```python
from build123d import *

# Parameters (mm, degrees)
SKETCH1_R           = 9.6
SKETCH1_R_2         = 4.2
BOSS_EXTRUDE1_DEPTH = 2
SKETCH4_W           = 58
SKETCH4_H           = 57.7
SKETCH4_R           = 2
SKETCH4_R_2         = 9.6
BOSS_EXTRUDE3_DEPTH = 2
SKETCH5_R           = 2
CUT_EXTRUDE1_DEPTH  = 4
SKETCH6_W           = 43
SKETCH6_H           = 57.7
SKETCH6_R           = 3.75
SKETCH6_R_2         = 9.6
SKETCH6_R_3         = 2
BOSS_EXTRUDE4_DEPTH = 5
CUT_EXTRUDE2_DEPTH  = 48.972101267
BOSS_EXTRUDE5_DEPTH = 6
BOSS_EXTRUDE6_DEPTH = 1.5


with BuildPart() as part:
    # Sketch1 → Boss-Extrude1 (new body)
    with BuildSketch(Plane.XY):
        with BuildLine():
            Line((38, 28.85), (20, 28.85))
            Line((20, 28.85), (20, 21.79369023))
            Line((20, 21.79369023), (17.201699017, 17.757141063))
            ThreePointArc((17.201699017, 17.757141063), (12.496432266, 16.141438171), (9.55, 20.15))
            Line((9.55, 20.15), (9.55, 28.85))
            Line((9.55, 28.85), (-9.55, 28.85))
            Line((-9.55, 28.85), (-9.55, 20.15))
            ThreePointArc((-9.55, 20.15), (-12.496432266, 16.141438171), (-17.201699017, 17.757141063))
            Line((-17.201699017, 17.757141063), (-20, 21.79369023))
            Line((-20, 21.79369023), (-20, -16.371914064))
            Line((-20, -16.371914064), (-16.312, -16.371914064))
            Line((-16.312, -16.371914064), (-12.349992933, -13.321914064))
            ThreePointArc((-12.349992933, -13.321914064), (-6.459906996, -14.088), (-7.225992933, -19.978085936))
            Line((-7.225992933, -19.978085936), (-11.188, -23.028085936))
            ThreePointArc((-11.188, -23.028085936), (-12.396848296, -23.676050863), (-13.75, -23.9))
            Line((-13.75, -23.9), (-20, -23.9))
            Line((-20, -23.9), (-20, -28.85))
            Line((-20, -28.85), (9.55, -28.85))
            Line((9.55, -28.85), (9.55, -19.7))
            ThreePointArc((9.55, -19.7), (12.496432266, -15.691438171), (17.201699017, -17.307141063))
            Line((17.201699017, -17.307141063), (20, -21.34369023))
            Line((20, -21.34369023), (20, -28.85))
            Line((20, -28.85), (38, -28.85))
            Line((38, -28.85), (38, 28.85))
        make_face()
        with Locations((0, 8.8)):
            Circle(SKETCH1_R, mode=Mode.SUBTRACT)
        with Locations((-5.725, -6.1)):
            Circle(SKETCH1_R_2, mode=Mode.SUBTRACT)
        with Locations((5.725, -6.1)):
            Circle(SKETCH1_R_2, mode=Mode.SUBTRACT)
    extrude(amount=BOSS_EXTRUDE1_DEPTH)

    # Sketch4 → Boss-Extrude3 (add)
    with BuildSketch(Plane.XY.offset(2)):
        with Locations((9, 0)):
            Rectangle(SKETCH4_W, SKETCH4_H)
        with Locations((13.75, -19.7)):
            Circle(SKETCH4_R, mode=Mode.SUBTRACT)
        with Locations((-13.75, 20.15)):
            Circle(SKETCH4_R, mode=Mode.SUBTRACT)
        with Locations((13.75, 20.15)):
            Circle(SKETCH4_R, mode=Mode.SUBTRACT)
        with Locations((-13.75, -19.7)):
            Circle(SKETCH4_R, mode=Mode.SUBTRACT)
        with Locations((0, 8.8)):
            Circle(SKETCH4_R_2, mode=Mode.SUBTRACT)
    extrude(amount=BOSS_EXTRUDE3_DEPTH)

    # Sketch5 → Cut-Extrude1 (cut)
    with BuildSketch(Plane.XY.offset(4)):
        with Locations((31, 15)):
            Circle(SKETCH5_R)
        with Locations((31, -15)):
            Circle(SKETCH5_R)
    extrude(amount=-CUT_EXTRUDE1_DEPTH, mode=Mode.SUBTRACT)

    # Sketch6 → Boss-Extrude4 (add)
    with BuildSketch(Plane.XY.offset(4)):
        with Locations((1.5, 0)):
            Rectangle(SKETCH6_W, SKETCH6_H)
        with Locations((-13.75, -19.7)):
            Circle(SKETCH6_R, mode=Mode.SUBTRACT)
        with Locations((0, 8.8)):
            Circle(SKETCH6_R_2, mode=Mode.SUBTRACT)
        with Locations((-13.75, 20.15)):
            Circle(SKETCH6_R, mode=Mode.SUBTRACT)
        with Locations((13.75, 20.15)):
            Circle(SKETCH6_R, mode=Mode.SUBTRACT)
        with Locations((13.75, -19.7)):
            Circle(SKETCH6_R_3, mode=Mode.SUBTRACT)
    extrude(amount=BOSS_EXTRUDE4_DEPTH)

    # Sketch7 → Cut-Extrude2 (cut, through all)
    with BuildSketch(Plane.XY.offset(4)):
        with BuildLine():
            Line((30.5, 28.85), (38, 28.85))
            Line((38, 28.85), (38, 21.35))
            ThreePointArc((38, 21.35), (35.803300859, 26.653300859), (30.5, 28.85))
        make_face()
        with BuildLine():
            Line((38, -28.85), (38, -21.35))
            ThreePointArc((38, -21.35), (35.803300859, -26.653300859), (30.5, -28.85))
            Line((30.5, -28.85), (38, -28.85))
        make_face()
    extrude(amount=-CUT_EXTRUDE2_DEPTH, mode=Mode.SUBTRACT)

    # Sketch9 → Boss-Extrude5 (add)
    with BuildSketch(Plane.ZY.offset(20)):
        Polygon((9, -28.85), (9, -40.85), (0, -40.85), (0, -35.15), (3, -35.15), (3, -28.85), align=None)
    extrude(amount=-BOSS_EXTRUDE5_DEPTH)

    # Sketch10 → Boss-Extrude6 (add)
    with BuildSketch(Plane.XY.offset(9)):
        Polygon((-14, -40.85), (-4, -40.85), (2.92820323, -28.85), (-14, -28.85), align=None)
    extrude(amount=-BOSS_EXTRUDE6_DEPTH)


solid = part.part
```
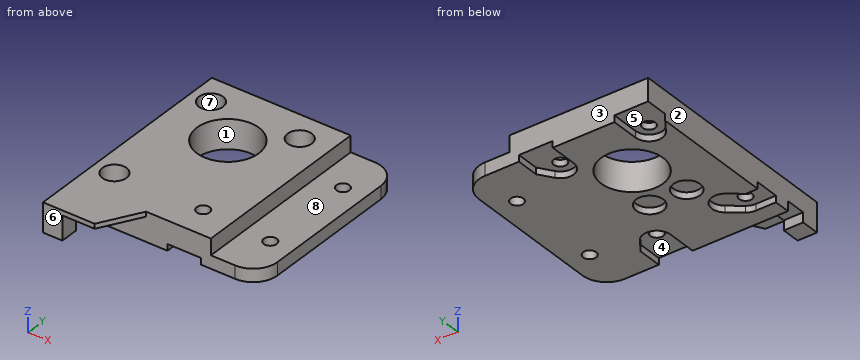
The listing builds one solid part. Answer for the finished solid, in the listing's coordinates (mm). Face numbers are marked on the shaded views. A direction names the side the tool comes from. Give positions to 0.01 mm unless a question says otherwise; leave off trailing zeros. Order: outer loops, then holes, each group sorted by start corner. A loop starts at its lowest first (then second) coordinate and runs counter-clockwise, first axis right, second up. Notation, with made-up numbers: (-19, 15) -> (17, 15) arc R20 ccw to (17, 24) -> close; hole circle Ø3 at (-32, 43.5). An arc over 180 degrees is marked (long way). Answer as CSV lines item,"result". Start each with the question number.
Q1. A cutting plane is placed at D-D (y = 1.5). Determine the outline of the cut face in (x, z), then the cut area to 3 significant figures.
Q2. Determine the mould class of the marked faces 1, 2 and 3 for opening direction Y: pulls with the +Y half, pulls with the -Y half, needs draft (parallel to the pull), parting line crosses it, or undercut.
Q3. Which of the six approach directions +Z, -Z, +X, -X, +Y, -Y give full straight-line access (tool end or side, diameter ignored) to the marked faces 4, 5, 6, 7 and 8?
Q4. A cutting plane is placed at C-C (y = -6.1). Determine the outline of the cut face in (x, z) (3 decimals), then the cut area to 3 significant figures.
Q5. A cutting plane is placed at A-A (x = 13.75). Determine the outline of the cut face in (y, z), then the cut area to 3 significant figures.
Q6. A cutting plane is placed at B-B (y = 8.8). Determine the outline of the cut face in (x, z).
Q7. Find the intervals of material crossed by L1, parallel to Y at x = -13.75, z = 7.3; L2, parallel to X at y = 20, z = 7.5; L3, parallel to Y at x = 13.75, z = 5.25, in increasing order.
Q8. Given pin 1 (1.6 mm diameter, centred on y = -22.5, z = 1.5, fed in from +X); pin 2 (2 mm diameter, centred on x = 14, y = 21.5, fed in from +Z); pin 3 (1.6 mm diameter, centred on y = 23.5, z = 0.5, fed in from +X), each flat-ended and moving along its own axis, determine where each tip first touches the part or whether it passes through.
Results found:
1,outline,"(-20, 0) -> (-6.23, 0) -> (-6.23, 9) -> (-20, 9) -> close; (6.23, 0) -> (38, 0) -> (38, 4) -> (23, 4) -> (23, 9) -> (6.23, 9) -> close"
1,area,"335 mm2"
2,face 1,"undercut"
2,face 2,"needs draft"
2,face 3,"pulls with the +Y half"
3,face 4,"-Z, -Y"
3,face 5,"-Z, +Y"
3,face 6,"+Z, -Z, +X, -X, -Y"
3,face 7,"+Z"
3,face 8,"+Z, +X, +Y, -Y"
4,outline,"(-20, 0) -> (-9.925, 0) -> (-9.925, 2) -> (-1.525, 2) -> (-1.525, 0) -> (1.525, 0) -> (1.525, 2) -> (9.925, 2) -> (9.925, 0) -> (38, 0) -> (38, 4) -> (23, 4) -> (23, 9) -> (-20, 9) -> close"
4,area,"413 mm2"
5,outline,"(-28.85, 2) -> (-21.7, 2) -> (-21.7, 9) -> (-28.85, 9) -> close; (-17.7, 2) -> (-15.5, 2) -> (-15.5, 0) -> (15.95, 0) -> (15.95, 2) -> (18.15, 2) -> (18.15, 4) -> (16.4, 4) -> (16.4, 9) -> (-17.7, 9) -> close; (22.15, 2) -> (28.85, 2) -> (28.85, 9) -> (23.9, 9) -> (23.9, 4) -> (22.15, 4) -> close"
5,area,"393 mm2"
6,outline,"(-20, 0) -> (-9.6, 0) -> (-9.6, 9) -> (-20, 9) -> close; (9.6, 0) -> (38, 0) -> (38, 4) -> (23, 4) -> (23, 9) -> (9.6, 9) -> close"
7,L1,"-28.85 to -23.45, -15.95 to 16.4, 23.9 to 28.85"
7,L2,"-20 to -17.5, -10 to 10, 17.5 to 23"
7,L3,"-28.85 to -21.7, -17.7 to 16.4, 23.9 to 28.85"
8,pin 1,"x = 37.99"
8,pin 2,"z = 4"
8,pin 3,"x = 37.88"
